Input: part model. Units: mm. Frame: model coordinates. A direction names the side the tool comes from. Coordinates: 2 decimals unless noted, no trailing zeros. Loops run counter-clockwise (first coordinate to the right, second up) from the corner with the lowest first, then second, coordinate; pieces in that order, holes last. Notation, with made-up numbers: (78, -22) - (92, -22) arc R25 ccw to (92, 0) - close; hole circle Ø7 at (-35.5, 66). An arc over 180 degrees is marked (long way). Use one line per item in the form item = value.
from build123d import *

# Parameters (mm, degrees)
SKETCH1_W             = 10
SKETCH1_H             = 13.5
SKETCH1_R             = 1.75
BOSS_EXTRUDE1_DEPTH   = 2.5
BOSS_EXTRUDE1_2_DEPTH = 2.5
BOSS_EXTRUDE2_DEPTH   = 1.5
SKETCH5_R             = 1.7499965
CUT_EXTRUDE1_DEPTH    = 12.446


with BuildPart() as part:
    # Sketch1 → Boss-Extrude1 (new body)
    with BuildSketch(Plane.XY):
        with Locations((8.63063628, 74.671921363)):
            Rectangle(SKETCH1_W, SKETCH1_H)
        with Locations((8.63063628, 74.421921363)):
            Circle(SKETCH1_R, mode=Mode.SUBTRACT)
    extrude(amount=BOSS_EXTRUDE1_DEPTH)



with BuildPart() as body_2:
    # Sketch1 → Boss-Extrude1 2 (new body)
    with BuildSketch(Plane.XY):
        with Locations((8.63063628, 59.171921363)):
            Rectangle(SKETCH1_W, SKETCH1_H)
        with Locations((8.63063628, 59.921921363)):
            Circle(SKETCH1_R, mode=Mode.SUBTRACT)
    extrude(amount=BOSS_EXTRUDE1_2_DEPTH)


with BuildPart() as part_1:
    add(part.part)

    add(body_2.part)  # Boss-Extrude2 merges body 2
    # Sketch2 → Boss-Extrude2 (add)
    with BuildSketch(Plane.ZY.offset(-3.63063628)):
        with BuildLine():
            Line((6.100159914, 65.921921363), (2.5, 65.921921363))
            Line((2.5, 65.921921363), (2.5, 52.421921363))
            Line((2.5, 52.421921363), (22.12, 67.921921363))
            Line((22.12, 67.921921363), (22.12, 73.801921363))
            ThreePointArc((22.12, 73.801921363), (19.888153673, 79.190075036), (14.5, 81.421921363))
            Line((14.5, 81.421921363), (2.5, 81.421921363))
            Line((2.5, 81.421921363), (2.5, 67.921921363))
            Line((2.5, 67.921921363), (6.100159914, 67.921921363))
            Line((6.100159914, 67.921921363), (6.100159914, 65.921921363))
        make_face()
    boss_extrude2 = extrude(amount=-BOSS_EXTRUDE2_DEPTH)

    # Mirror1: Boss-Extrude2 across plane
    add(boss_extrude2.mirror(Plane.ZY.offset(-8.63063628)))

    # Sketch5 → Cut-Extrude1 (cut)
    with BuildSketch(Plane.ZY.offset(-3.63063628)):
        with Locations(Location((14.5, 73.801921363, 0), (0, 0, 270))):
            Circle(SKETCH5_R)
    extrude(amount=-CUT_EXTRUDE1_DEPTH, mode=Mode.SUBTRACT)


solid = part_1.part
Q1. Pull-direction query (Y, two-part tool) for faces 4 (the flat face through (13, 67, 6.1)), 5 (the flat face through (12.89, 60.06, 12.17)), 6 (the flat face through (3.631, 70, 8)); classes: pulls with the +Y half, pulls with the -Y half, needs draft (parallel to the pull), parting line crosses it, or undercut.
Check values:
face_4 = undercut
face_5 = pulls with the -Y half
face_6 = needs draft
Q2. Cut plane A-A, the plane x = 5.75. Return loops of the section in (y, z).
Check values:
outline = (52.42, 0) - (65.92, 0) - (65.92, 2.5) - (52.42, 2.5) - close; (67.92, 0) - (81.42, 0) - (81.42, 2.5) - (67.92, 2.5) - close
Q3. First-contact query: P1, Ø2, axis at y = 73.8, z = 14.5, coming from the +X side; P2, Ø3, axis at x = 5.5, y = 77.5, coming from the +Z side; P3, Ø4, axis at x = 5.5, z = 16.5, coming from the -Y side; P4, Ø2, axis at x = 7, y = 66.5, coming from the +Z side. Flat tips, straight axial feed; report the tip coordinate or a pass-through.
Check values:
P1 = through
P2 = 21.78
P3 = 61.93
P4 = 2.5
Q4. Cut plane C-C, the plane x = 7.25. Return loops of the section in (y, z), then the cut area to 3 significant figures.
Check values:
outline = (52.42, 0) - (58.85, 0) - (58.85, 2.5) - (52.42, 2.5) - close; (61, 0) - (65.92, 0) - (65.92, 2.5) - (61, 2.5) - close; (67.92, 0) - (73.35, 0) - (73.35, 2.5) - (67.92, 2.5) - close; (75.5, 0) - (81.42, 0) - (81.42, 2.5) - (75.5, 2.5) - close
area = 56.7 mm²
Q5. Cut plane B-B, the plane z = 20. Return loops of the section in (x, y), then the cut area to 3 significant figures.
Check values:
outline = (3.63, 66.25) - (5.13, 66.25) - (5.13, 79.08) - (3.63, 79.08) - close; (12.13, 66.25) - (13.63, 66.25) - (13.63, 79.08) - (12.13, 79.08) - close
area = 38.5 mm²
Q6. Cut plane D-D, the plane y = 60.5. Return loops of the section in (x, z), then the cut area to 3 significant figures.
Check values:
outline = (3.63, 0) - (6.98, 0) - (6.98, 2.5) - (5.13, 2.5) - (5.13, 12.73) - (3.63, 12.73) - close; (10.28, 0) - (13.63, 0) - (13.63, 12.73) - (12.13, 12.73) - (12.13, 2.5) - (10.28, 2.5) - close
area = 47.4 mm²
Q7. Set-up query: faces 1 (the cylindrical face through (12.87, 75.55, 14.58)), 2 (the flat face through (9, 65.922, 2)), 3 (the flat face through (5.131, 70, 12)). Return all of +Z, -Z, +X, -X, +Y, -Y with unobstructed straight access to the full face (end or side cutting, diameter ignored); none if empty.
Check values:
face_1 = +X, -X
face_2 = -Z, +X, -X
face_3 = +Z, +Y, -Y
Q8. Ray query, line 1 along X through (y, z) = (64, 6.25); line 2 along Z through (x, y) = (6, 62.25); line 3 along X through (y, z) = (61.5, 1.75). Return the intervals inside material, ascending. Write a range as [from, to].
Check values:
line_1 = [3.63, 5.13], [12.13, 13.63]
line_2 = [0, 2.5]
line_3 = [3.63, 7.87], [9.39, 13.63]
